```python
from build123d import *

# Parameters (mm, degrees)
SKETCH_1_R          = 15
EXTRUDE_1_DEPTH     = 32
CHAMFER_1_SIZE      = 2
SKETCH_2_R          = 16
EXTRUDE_2_DEPTH     = 26
SKETCH_3_R          = 19
EXTRUDE_3_DEPTH     = 13
SKETCH_4_R          = 14
EXTRUDE_4_DEPTH     = 1.5
SKETCH_5_R          = 15
EXTRUDE_5_DEPTH     = 14.5
SKETCH_6_R          = 14
EXTRUDE_6_DEPTH     = 23
SKETCH_7_R          = 12
EXTRUDE_7_DEPTH     = 34
FILLET_1_R          = 1.5
CHAMFER_2_SIZE      = 2
CUT_EXTRUDE_START   = 16
CUT_EXTRUDE_1_DEPTH = 6
CUT_EXTRUDE_START_2 = 12
CUT_EXTRUDE_2_DEPTH = 3.5


with BuildPart() as part:
    # Sketch 1 → Extrude 1 (new body)
    with BuildSketch(Plane(origin=(0, 0, 0), x_dir=(0, 0, -1), z_dir=(1, 0, 0))):
        Circle(SKETCH_1_R)
    extrude(amount=EXTRUDE_1_DEPTH)

    # Chamfer 1
    chamfer_1_edges = [part.edges().sort_by_distance(p)[0] for p in [
        (0, 0, 15),
    ]]
    chamfer(chamfer_1_edges, length=CHAMFER_1_SIZE)

    # Sketch 2 → Extrude 2 (add)
    with BuildSketch(Plane(origin=(32, 0, 0), x_dir=(0, 0, -1), z_dir=(1, 0, 0))):
        with Locations(Location((0, 0, 0), (0, 0, 180))):
            Circle(SKETCH_2_R)
    extrude(amount=EXTRUDE_2_DEPTH)

    # Sketch 3 → Extrude 3 (add)
    with BuildSketch(Plane(origin=(58, 0, 0), x_dir=(0, 0, -1), z_dir=(1, 0, 0))):
        with Locations(Location((0, 0, 0), (0, 0, 180))):
            Circle(SKETCH_3_R)
    extrude(amount=EXTRUDE_3_DEPTH)

    # Sketch 4 → Extrude 4 (add)
    with BuildSketch(Plane(origin=(71, 0, 0), x_dir=(0, 0, -1), z_dir=(1, 0, 0))):
        Circle(SKETCH_4_R)
    extrude(amount=EXTRUDE_4_DEPTH)

    # Sketch 5 → Extrude 5 (add)
    with BuildSketch(Plane(origin=(72.5, 0, 0), x_dir=(0, 0, -1), z_dir=(1, 0, 0))):
        Circle(SKETCH_5_R)
    extrude(amount=EXTRUDE_5_DEPTH)

    # Sketch 6 → Extrude 6 (add)
    with BuildSketch(Plane(origin=(87, 0, 0), x_dir=(0, 0, -1), z_dir=(1, 0, 0))):
        Circle(SKETCH_6_R)
    extrude(amount=EXTRUDE_6_DEPTH)

    # Sketch 7 → Extrude 7 (add)
    with BuildSketch(Plane(origin=(110, 0, 0), x_dir=(0, 0, -1), z_dir=(1, 0, 0))):
        Circle(SKETCH_7_R)
    extrude(amount=EXTRUDE_7_DEPTH)

    # Fillet 1
    fillet_1_edges = [part.edges().sort_by_distance(p)[0] for p in [
        (110, 0, 12),
    ]]
    fillet(fillet_1_edges, radius=FILLET_1_R)

    # Chamfer 2
    chamfer_2_edges = [part.edges().sort_by_distance(p)[0] for p in [
        (144, 0, 12),
    ]]
    chamfer(chamfer_2_edges, length=CHAMFER_2_SIZE)

    # Sketch 8 → Cut-Extrude 1 (cut)
    with BuildSketch(Plane(origin=(0, 0, 0), x_dir=(1, 0, 0), z_dir=(0, 1, 0)).offset(CUT_EXTRUDE_START)):
        with BuildLine():
            Line((39, 5), (51, 5))
            ThreePointArc((51, 5), (56, 0), (51, -5))
            Line((51, -5), (39, -5))
            ThreePointArc((39, -5), (34, 0), (39, 5))
        make_face()
    extrude(amount=-CUT_EXTRUDE_1_DEPTH, mode=Mode.SUBTRACT)

    # Sketch 9 → Cut-Extrude 2 (cut)
    with BuildSketch(Plane(origin=(0, 0, 0), x_dir=(1, 0, 0), z_dir=(0, 1, 0)).offset(CUT_EXTRUDE_START_2)):
        with BuildLine():
            Line((117, 4), (134, 4))
            ThreePointArc((134, 4), (138, 0), (134, -4))
            Line((134, -4), (117, -4))
            ThreePointArc((117, -4), (113, 0), (117, 4))
        make_face()
    extrude(amount=-CUT_EXTRUDE_2_DEPTH, mode=Mode.SUBTRACT)


solid = part.part
```
The listing builds one solid part. Answer for the finished solid, in the listing's coordinates (mm). A direction names the side the tool comes from. Give positions to 0.01 mm unless a question says otherwise; leave off trailing zeros. Order: outer loops, then holes, each group sorted by start corner. A loop starts at its lowest first (then second) coordinate and runs counter-clockwise, first axis right, second up. Notation, with made-up numbers: (-31, 58.5) - (8, 58.5) arc R24 ccw to (8, 76.5) - close; hole circle Ø10 at (-38, 79.5). An arc over 180 degrees is marked (long way). Answer in a Markdown table with one row per item. Add a question column.
Q1. Given P1, Ø1.6, axis at x = 44, y = 14, coming from the -Z side; P2, Ø6.5, axis at x = 121.5, z = 1.5, coming from the +Y side; P3, Ø6, axis at y = -6.5, z = 2, coming from the -X side; P4, Ø1, axis at x = 27, z = -11, coming from the +Y side, each flat-ended and moving along its own axis, determine where each tip first touches the part or whether it passes through.
Q2. For a pull along Z with two mould halves and no side action, classify faces 1 (the cylindrical face through (34, 13, 0)), 2 (the cylindrical face through (16.79, 0.66, 14.985)), 3 (the flat face through (71, 11, -9)), 4 (the flat face through (45, 13, -5)) as released by +Z, released by -Z, zero draft, split by the parting line, or undercut.
Q3. The part is cut by section C-C (x = 16). Determine the outline of the cut face in (y, z), then the cut area to 3 significant figures.
Q4. Which of the six approach directions +Z, -Z, +X, -X, +Y, -Y give full straight-line access (tool end or side, diameter ignored) to faces 5 (the cylindrical face through (44.82, -13.49, 8.6)), 6 (the cylindrical face through (126.536, -11.715, 2.601)), 7 (the cylindrical face through (56, 13, 0)), 8 (the cylindrical face through (71.74, -5.362, -12.932)), 9 (the flat face through (144, 0, 0))?
Q5. Find the intervals of material crossed by line 1 along Z through (x, y) = (17, -0.5); line 2 along X through (y, z) = (1, 16); line 3 along Z through (x, y) = (35.5, 13.5), in increasing order. Write a range as [from, to].
Q6. The part is cut by section D-D (z = 17.5). Determine the outline of the cut face in (x, y).
Q7. The part is cut by section B-B (x = 61). Determine the outline of the cut face in (y, z), then the cut area to 3 significant figures.
Determined:
| question | item | result |
|---|---|---|
| 1 | P1 | stops at z = -9.04 |
| 1 | P2 | stops at y = 11.31 |
| 1 | P3 | stops at x = 0 |
| 1 | P4 | stops at y = 10.71 |
| 2 | face 1 | undercut |
| 2 | face 2 | split by the parting line |
| 2 | face 3 | zero draft |
| 2 | face 4 | undercut |
| 3 | outline | circle Ø30 at (0, 0) |
| 3 | area | 707 mm² |
| 4 | face 5 | -X |
| 4 | face 6 | +X |
| 4 | face 7 | +Y |
| 4 | face 8 | none |
| 4 | face 9 | +Z, -Z, +X, +Y, -Y |
| 5 | line 1 | z = [-14.99, 14.99] |
| 5 | line 2 | x = [58, 71] |
| 5 | line 3 | z = [-8.59, -3.57], [3.57, 8.59] |
| 6 | outline | (58, -7.4) - (71, -7.4) - (71, 7.4) - (58, 7.4) - close |
| 7 | outline | circle Ø38 at (0, 0) |
| 7 | area | 1,130 mm² |
